Build history of the part. All positions in model axes, mm. Face numbers are marked on the shaded views. A direction names the side the tool comes from. Give positions to 0.01 mm unless a question says otherwise; leave off trailing zeros. Loops run counter-clockwise (first coordinate to the right, second up) from the corner with the lowest first, then second, coordinate; pieces in that order, holes last.
1) Band-saw the part on B-B on y = 1.7. List the corners of the cut face in (x, z), then the cut area to 3 significant figures.
2) Two-plate mould, pull along Y, no slides. Class the marked faces 1, 2 and 3: +Y half, -Y half, draft (parallel to the pull), parting line (faces both ways), or undercut.
3) 3-axis set-ups, long thin cutter, end or side, ignore diameter. For the marked faces 4, 5 and 6: which of +Z, -Z, +X, -X, +Y, -Y reach the whole face in a straight line?
4) Wall check: line 1 (Y direction, x = 1.25, z = 2.85); line 2 (X direction, y = 2.25, z = 1.85); line 3 (Y direction, x = 2.25, z = 2.55). Give the ranges that are in metal, low to high.
5) Band-saw the part on A-A on z = 4.4. List the corners of the cut face in (x, y).
6) Flat gauge pins, fed straight in: P1, Ø1.5, axis at y = 0.5, z = 1.5, coming from the +X side; P2, Ø1, axis at x = -0.5, z = 4, coming from the +Y side. Where does each tip first touch, or does it go through?
7) Band-saw the part on D-D on x = 2.25. List the corners of the cut face in (y, z), then the cut area to 3 significant figures.
8) Band-saw the part on C-C on z = 0.8. List the corners of the cut face in (x, y), then the cut area to 3 significant figures.
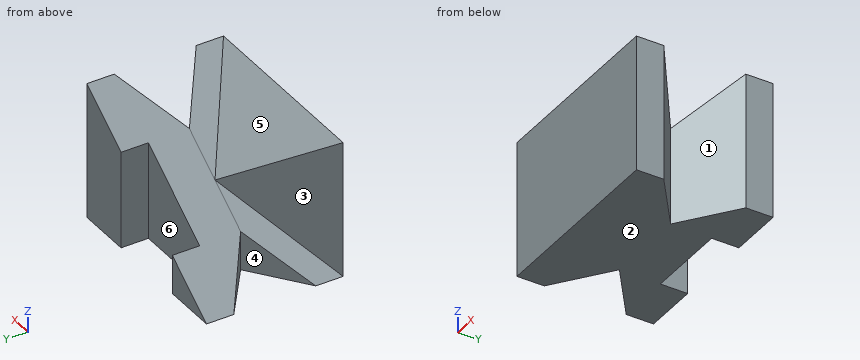
```python
from build123d import *

# Parameters (mm, degrees)
BOSS_EXTRUDE1_DEPTH = 5
CUT_EXTRUDE1_DEPTH  = 5
BOSS_EXTRUDE2_DEPTH = 2.5
CUT_EXTRUDE2_DEPTH  = 2.5
CUT_EXTRUDE3_DEPTH  = 2.5


with BuildPart() as part:
    # Sketch1 → Boss-Extrude1 (new body)
    with BuildSketch(Plane.XY):
        Polygon((-3.5, -2.5), (3.5, -2.5), (3.5, -1.5), (1.5, 0), (3.5, 1.5), (3.5, 2.5), (1.5, 2.5), (1.5, 1.5), (-1.5, 1.5), (-1.5, 2.5), (-3.5, 2.5), (-3.5, 1.5), (-1.5, 0), (-3.5, -1.5), align=None)
    extrude(amount=BOSS_EXTRUDE1_DEPTH)

    # Sketch2 → Cut-Extrude1 (cut)
    with BuildSketch(Plane(origin=(0, 2.5, 0), x_dir=(1, 0, 0), z_dir=(0, 1, 0))):
        Polygon((-3.5, 0), (3.5, -5), (-3.5, -5), align=None)
    extrude(amount=-CUT_EXTRUDE1_DEPTH, mode=Mode.SUBTRACT)

    # Sketch3 → Boss-Extrude2 (add)
    with BuildSketch(Plane.XZ.offset(2.5)):
        Polygon((-3.5, 0), (-3.5, 5), (3.5, 5), align=None)
    extrude(amount=-BOSS_EXTRUDE2_DEPTH)

    # 3DSketch2 → Cut-Extrude2 (cut, along a direction that is not the sketch's normal)
    with BuildSketch(Plane(origin=(-3.5, -2.5, 0), x_dir=(0, 0, 1), z_dir=(-0.5812381937190964, 0.8137334712067351, 0))):
        Polygon((0, 0), (2.5, 4.301162634), (5, 0), align=None)
    extrude(amount=CUT_EXTRUDE2_DEPTH, dir=(0, 1, 0), mode=Mode.SUBTRACT)

    # 3DSketch3 → Cut-Extrude3 (cut, along a direction that is not the sketch's normal)
    with BuildSketch(Plane(origin=(0, 0, 2.5), x_dir=(-0.7035264706814485, -0.502518907629606, 0.502518907629606), z_dir=(0, 0.7071067811865476, 0.7071067811865476))):
        Polygon((0, 0), (4.974937186, 0), (0.050251891, 4.974683382), align=None)
    extrude(amount=CUT_EXTRUDE3_DEPTH, dir=(0, 1, 0), mode=Mode.SUBTRACT)


solid = part.part
```
Findings below:
1. outline: (-3.5, 0) - (-1.5, 0) - (-1.5, 1.43) - close; (1.5, 0) - (3.5, 0) - (3.5, 5) - (1.5, 3.57) - close
1. area: 10.0 mm2
2. face 1: undercut
2. face 2: draft
2. face 3: +Y half
3. face 4: +Z, -Z, -X
3. face 5: +Z, -X, +Y
3. face 6: +Z, -Z, +Y
4. line 1: y = -2.5 to 1.5
4. line 2: x = 1.5 to 3.5
4. line 3: y = -2.5 to -0.56, 0.56 to 2.5
5. outline: (-3.5, -2.5) - (3.5, -2.5) - (3.5, -1.5) - (2.66, -0.87) - (2.66, -1.9) - (-2.66, -1.9) - close; (2.66, 0.87) - (3.5, 1.5) - (3.5, 2.5) - (2.66, 2.5) - close
6. P1: stops at x = 3.17
6. P2: stops at y = -1
7. outline: (-2.5, 0) - (-0.56, 0) - (-0.56, 4.11) - (-1.61, 4.11) - (-2.5, 5) - close; (0.56, 0) - (2.5, 0) - (2.5, 4.11) - (0.56, 4.11) - close
7. area: 16.3 mm2
8. outline: (-3.5, -2.5) - (3.5, -2.5) - (3.5, -1.5) - (1.5, 0) - (3.5, 1.5) - (3.5, 2.5) - (1.5, 2.5) - (1.5, 1.5) - (-1.5, 1.5) - (-1.5, 2.5) - (-2.38, 2.5) - (-2.38, 0.66) - (-1.5, 0) - (-2.38, -0.66) - (-2.38, -1.7) - close
8. area: 23.3 mm2
